Part model, mm, in its own coordinate system. A direction names the side the tool comes from. Round coordinates to 2 decimals unless told otherwise and drop trailing zeros. Order: outer loops, then holes, each group sorted by start corner. A loop starts at its lowest first (then second) coordinate and runs counter-clockwise, first axis right, second up. Notation, with made-up numbers: (37, 83) -> (96, 83) arc R11 cw to (96, 102) -> close; hole circle Ø3 at (11.25, 23.25). An arc over 180 degrees is marked (long way). Use CSV: the item, a comma, the result in double quotes.
```python
from build123d import *

# Parameters (mm, degrees)
SKETCH004_W     = 50
SKETCH004_H     = 182
PAD003_DEPTH    = 6
PAD010_DEPTH    = 20
SKETCH015_R     = 1.6
POCKET_DEPTH    = 20
PAD_DEPTH       = 12
PAD018_DEPTH    = 12
SKETCH019_R     = 1.7
HOLE_DEPTH      = 40
CHAMFER002_SIZE = 2
CHAMFER_SIZE    = 3


with BuildPart() as part:
    # Sketch004 → Pad003 (new body)
    with BuildSketch(Plane.XY):
        with Locations((0, -69)):
            Rectangle(SKETCH004_W, SKETCH004_H)
        with BuildLine():
            ThreePointArc((-16, -134), (0, -150), (16, -134))
            Line((16, -134), (16, 0))
            ThreePointArc((16, 0), (0, 16), (-16, 0))
            Line((-16, -134), (-16, 0))
        make_face(mode=Mode.SUBTRACT)
    extrude(amount=PAD003_DEPTH)

    # Sketch016 → Pad010 (join)
    with BuildSketch(Plane.XY):
        with BuildLine():
            ThreePointArc((-11.5, 15), (-17.5, 21), (-23.5, 15))
            Line((-23.5, 15), (-23.5, 6.359301))
            ThreePointArc((-23.5, 6.359301), (-17.5, 0.359301), (-11.5, 6.359301))
            Line((-11.5, 15), (-11.5, 6.359301))
        make_face()
        with BuildLine():
            ThreePointArc((23.5, 15), (17.5, 21), (11.5, 15))
            Line((11.5, 15), (11.5, 6.359301))
            ThreePointArc((11.5, 6.359301), (17.5, 0.359301), (23.5, 6.359301))
            Line((23.5, 15), (23.5, 6.359301))
        make_face()
    extrude(amount=PAD010_DEPTH)

    # Sketch015 → Pocket (cut)
    with BuildSketch(Plane.XY):
        with Locations((-17.5, 14)):
            Circle(SKETCH015_R)
        with Locations((17.5, 14)):
            Circle(SKETCH015_R)
    extrude(amount=POCKET_DEPTH, mode=Mode.SUBTRACT)

    # Sketch018 → Pad (join)
    with BuildSketch(Plane.XZ.offset(148)):
        Polygon((-16.5, 0), (16.5, 0), (30.504151, 20), (42.504151, 20), (42.504151, 24), (29.103736, 24), (16.5, 6), (-16.5, 6), (-29.103736, 24), (-42.504151, 24), (-42.504151, 20), (-30.504151, 20), align=None)
    extrude(amount=PAD_DEPTH)

    # Sketch034 → Pad018 (join)
    with BuildSketch(Plane.XZ.offset(55)):
        Polygon((-16.5, 0), (16.5, 0), (30.504151, 20), (42.504151, 20), (42.504151, 24), (29.103736, 24), (16.5, 6), (-16.5, 6), (-29.103736, 24), (-42.504151, 24), (-42.504151, 20), (-30.504151, 20), align=None)
    extrude(amount=PAD018_DEPTH)

    # Sketch019 → Hole (cut)
    with BuildSketch(Plane.XY):
        with Locations((-36.5, -154)):
            Circle(SKETCH019_R)
        with Locations((36.5, -154)):
            Circle(SKETCH019_R)
        with Locations((-36.5, -61)):
            Circle(SKETCH019_R)
        with Locations((36.5, -61)):
            Circle(SKETCH019_R)
    extrude(amount=HOLE_DEPTH, mode=Mode.SUBTRACT)

    # Chamfer002
    chamfer002_edges = [part.edges().sort_by_distance(p)[0] for p in [
        (-42.504151, -160, 22),
        (-42.504151, -148, 22),
        (42.504151, -160, 22),
        (42.504151, -148, 22),
        (-42.504151, -67, 22),
        (-42.504151, -55, 22),
        (42.504151, -67, 22),
        (42.504151, -55, 22),
    ]]
    chamfer(chamfer002_edges, length=CHAMFER002_SIZE)

    # Chamfer
    chamfer_edges = [part.edges().sort_by_distance(p)[0] for p in [
        (-25, -160, 3),
        (25, -160, 3),
        (25, 22, 3),
        (-25, 22, 3),
    ]]
    chamfer(chamfer_edges, length=CHAMFER_SIZE)


solid = part.part
```
(1) Probe probe 1 along Y at (x, z) = (36.5, 22.6); probe 2 along X at (y, z) = (-154, 22.9); probe 3 along X at (y, z) = (-61, 22.3). List the from-to ranges inside material, lowest first. Write a range as [from, to].
Reply:
probe 1,"[-160, -155.7], [-152.3, -148], [-67, -62.7], [-59.3, -55]"
probe 2,"[-42.5, -38.2], [-34.8, -28.33], [28.33, 34.8], [38.2, 42.5]"
probe 3,"[-42.5, -38.2], [-34.8, -27.91], [27.91, 34.8], [38.2, 42.5]"
(2) Drop flat-ended pins along their axis: P1, Ø6, axis at y = -1, z = 5, coming from the -X side; P2, Ø9.5, axis at x = 36, y = -154.5, coming from the -Z side; P3, Ø9.5, axis at y = 10, z = 10, coming from the +X side. Give the stop position or say it passes through.
Reply:
P1,"x = -25"
P2,"z = 20"
P3,"x = 25"
(3) Pull direction Z, two halves, no side cores. Call faces 4 (the face through (28, -67, 18)), 5 (the face through (-34, -154, 24)), 6 (the face through (25.534, -60.916, 12.902)): released by +Z, released by -Z, zero draft, split by the parting line, or undercut.
Reply:
face 4,"zero draft"
face 5,"released by +Z"
face 6,"undercut"
(4) Cut at C-C, the plane x = 33. Give the cut face in (y, z).
Reply:
outline,"(-160, 20) -> (-148, 20) -> (-148, 24) -> (-160, 24) -> close; (-67, 20) -> (-55, 20) -> (-55, 24) -> (-67, 24) -> close"
(5) Cut at A-A, the plane y = -9.5. Give the cut face in (x, z).
Reply:
outline,"(-25, 0) -> (-16, 0) -> (-16, 6) -> (-25, 6) -> close; (16, 0) -> (25, 0) -> (25, 6) -> (16, 6) -> close"
(6) Cut at D-D, the plane z = 4. Give the cut face in (x, y), then the cut area to 3 significant figures.
Reply:
outline,"(-25, -157) -> (-22, -160) -> (22, -160) -> (25, -157) -> (25, 19) -> (22, 22) -> (-22, 22) -> (-25, 19) -> close; hole circle Ø3.2 at (-17.5, 14); hole (-16, -134) arc R16 ccw to (-7.75, -148) -> (7.75, -148) arc R16 ccw to (16, -134) -> (16, -67) -> (-16, -67) -> close; hole (-16, -55) -> (16, -55) -> (16, 0) arc R16 ccw to (15.99, 0.55) arc R6 cw to (11.5, 6.36) -> (11.5, 11.12) arc R16 ccw to (-11.5, 11.12) -> (-11.5, 6.36) arc R6 cw to (-15.99, 0.55) arc R16 ccw to (-16, 0) -> close; hole circle Ø3.2 at (17.5, 14)"
area,"4,430 mm2"
(7) Cut at B-B, the plane z = 11.25. Give the cut face in (x, y), then the cut area to 3 significant figures.
Reply:
outline,"(-24.38, -160) -> (-20.18, -160) -> (-20.18, -148) -> (-24.38, -148) -> close; (-24.38, -67) -> (-20.18, -67) -> (-20.18, -55) -> (-24.38, -55) -> close; (-23.5, 6.36) arc R6 ccw to (-11.5, 6.36) -> (-11.5, 15) arc R6 ccw to (-23.5, 15) -> close; (11.5, 6.36) arc R6 ccw to (23.5, 6.36) -> (23.5, 15) arc R6 ccw to (11.5, 15) -> close; (20.18, -160) -> (24.38, -160) -> (24.38, -148) -> (20.18, -148) -> close; (20.18, -67) -> (24.38, -67) -> (24.38, -55) -> (20.18, -55) -> close; hole circle Ø3.2 at (-17.5, 14); hole circle Ø3.2 at (17.5, 14)"
area,"619 mm2"
(8) Which spindle directions (+Z, -Z, +X, -X, +Y, -Y) get a long thin tool onto all of the face, cutting with end or side? Do faces 1 (the face through (11.5, 11, 12)), 2 (the face through (-16, -101, 3)), 3 (the face through (23.5, 11, 13)). Say none if no direction does.
Reply:
face 1,"+Z"
face 2,"+Z, -Z"
face 3,"+Z, +X, +Y"
